```python
from build123d import *

# Parameters (mm, degrees)
SKETCH_W        = 80
SKETCH_H        = 47
PAD_DEPTH       = 4
SKETCH001_R     = 2.1
POCKET_DEPTH    = 4.001
SKETCH002_W     = 20
SKETCH002_H     = 16
PAD001_DEPTH    = 20
SKETCH003_R     = 1.6
POCKET001_DEPTH = 223.177811
POCKET002_DEPTH = 223.177811
CHAMFER_SIZE    = 3
CHAMFER_FACE9_W = 80
CHAMFER_FACE9_H = 4
POCKET003_DEPTH = 15.5
FILLET_R        = 4
FILLET001_R     = 1
SKETCH005_W     = 15
SKETCH005_H     = 16
POCKET004_DEPTH = 9
FILLET002_R     = 10


with BuildPart() as part:
    # Sketch → Pad (new body)
    with BuildSketch(Plane.XY):
        Rectangle(SKETCH_W, SKETCH_H)
    extrude(amount=PAD_DEPTH)

    # Sketch001 (on Face6 of Pad) → Pocket (cut, through all)
    with BuildSketch(Plane.XY.offset(4)):
        with Locations((-19, 19)):
            Circle(SKETCH001_R)
        with Locations((19, 19)):
            Circle(SKETCH001_R)
        with Locations((19, -19)):
            Circle(SKETCH001_R)
        with Locations((-19, -19)):
            Circle(SKETCH001_R)
    extrude(amount=-POCKET_DEPTH, mode=Mode.SUBTRACT)

    # Sketch002 (on Face5 of Pocket) → Pad001 (join)
    with BuildSketch(Plane.XY.offset(4)):
        with Locations((-30, 0)):
            Rectangle(SKETCH002_W, SKETCH002_H)
    pad001 = extrude(amount=PAD001_DEPTH)

    # Mirrored: Pad001 across YZ
    add(pad001.mirror(Plane.YZ))

    # Sketch003 (on Face15 of Mirrored) → Pocket001 (cut, through all)
    with BuildSketch(Plane.XZ.offset(8)):
        with Locations((-36, 8)):
            Circle(SKETCH003_R)
    pocket001 = extrude(amount=-POCKET001_DEPTH, mode=Mode.SUBTRACT)

    # Mirrored001: Pocket001 across YZ
    add(pocket001.mirror(Plane.YZ), mode=Mode.SUBTRACT)

    # Sketch004 (on Face15 of Mirrored001) → Pocket002 (cut, through all)
    with BuildSketch(Plane.XZ.offset(8)):
        with BuildLine():
            ThreePointArc((-40, 24), (-31.691484, 12.308516), (-20, 4))
            Line((-20, 24), (-20, 4))
            Line((-40, 24), (-20, 24))
        make_face()
    pocket002 = extrude(amount=-POCKET002_DEPTH, mode=Mode.SUBTRACT)

    # Mirrored002: Pocket002 across Sketch004 V_Axis
    add(pocket002.mirror(Plane(origin=(0, -8, 0), x_dir=(0, -1, 0), z_dir=(1, 0, 0))), mode=Mode.SUBTRACT)

    # Chamfer
    chamfer_edges = [part.edges().sort_by_distance(p)[0] for p in [
        (-40, 0, 24),
        (40, 0, 24),
    ]]
    chamfer(chamfer_edges, length=CHAMFER_SIZE)

    # Chamfer Face9 → Pocket003 (cut)
    with BuildSketch(Plane(origin=(0, -23.5, 2), x_dir=(-1, 0, 0), z_dir=(0, -1, 0))):
        Rectangle(CHAMFER_FACE9_W, CHAMFER_FACE9_H)
    extrude(amount=-POCKET003_DEPTH, mode=Mode.SUBTRACT)

    # Fillet
    fillet_edges = [part.edges().sort_by_distance(p)[0] for p in [
        (-40, 23.5, 2),
        (40, 23.5, 2),
    ]]
    fillet(fillet_edges, radius=FILLET_R)

    # Fillet001
    fillet001_edges = [part.edges().sort_by_distance(p)[0] for p in [
        (40, 13.75, 4),
    ]]
    fillet(fillet001_edges, radius=FILLET001_R)

    # Sketch005 (on DatumPlane) → Pocket004 (cut)
    with BuildSketch(Plane.XY.offset(10)):
        with Locations((-25.5, 0)):
            Rectangle(SKETCH005_W, SKETCH005_H)
    pocket004 = extrude(amount=POCKET004_DEPTH, mode=Mode.SUBTRACT)

    # Mirrored003: Pocket004 across Sketch005 V_Axis
    add(pocket004.mirror(Plane(origin=(0, 0, 10), x_dir=(0, 0, 1), z_dir=(1, 0, 0))), mode=Mode.SUBTRACT)

    # Fillet002
    fillet002_edges = [part.edges().sort_by_distance(p)[0] for p in [
        (33, 0, 13.675937),
        (29.19265, 0, 10),
        (-33, 0, 13.675937),
        (-29.19265, 0, 10),
    ]]
    fillet(fillet002_edges, radius=FILLET002_R)


solid = part.part
```
Design review of the part built by this model. Coordinates are the model's own, in mm. A direction names the side the tool comes from. Give positions to 0.01 mm unless a question says otherwise; leave off trailing zeros. Order: outer loops, then holes, each group sorted by start corner. A loop starts at its lowest first (then second) coordinate and runs counter-clockwise, first axis right, second up. Notation, with made-up numbers: (43, 31.25) - (51, 31.25) arc R7 cw to (51, 38.25) - close; hole circle Ø7 at (78.5, 55). An arc over 180 degrees is marked (long way). Use a Markdown table: item, result. Add a question column.
(1) Add section B-B on z = 11.75. Give the boundary of the cut face in (x, y), then the cut area to 3 significant figures.
(2) Machinability: for faces 1 (the face through (21.003, 19.631, 2.028)), 2 (the face through (29.51, -0.11, 9.49)), which of the approach directions +Z, -Z, +X, -X, +Y, -Y give a long, thin tool a straight path to every point of the face, cutting with its end or side? Answer none if there is none.
(3) Add section D-D on x = -16. Give the boundary of the cut face in (y, z).
(4) Mouldability with a two-part tool opening along Z and no side actions: class faces 3 (the face through (0, -8, 3)), 4 (the face through (-1, 11, 4)), 5 (the face through (-36.35, -0.11, 6.44)) as +Z half, -Z half, draft (parallel to the pull), parting line (faces both ways), or undercut.
(5) Add section C-C on y = 15. Give the boundary of the cut face in (x, z), then the cut area to 3 significant figures.
(6) Add section A-A on y = -1. Give the number of separate pieces and of enclosed holes in the cut face, then the cut area to 3 significant figures.
(7) Clearance check with flat-ended pins moving along their axes: P1, Ø2, axis at y = 8.5, z = 11, coming from the +X side; P2, Ø3.5, axis at x = 36, z = 8, coming from the +Y side; P3, Ø4, axis at x = -24, y = 20, coming from the +Z side. State where each tip first meets the part, or that it passes through.
(8) Wall thickness on probe 1 along X at (y, z) = (0.5, 8.5); probe 2 along Z at (x, y) = (36.5, 10.5); probe 3 along Y at (x, z) = (-27, 7.25): over which ranges is each line inside the solid? List them lowest first. Write a range as [from, to].
Report:
| question | item | result |
|---|---|---|
| 1 | outline | (-40, -8) - (-33.15, -8) - (-33.15, 8) - (-40, 8) - close; (33.15, -8) - (40, -8) - (40, 8) - (33.15, 8) - close |
| 1 | area | 219 mm² |
| 2 | face 1 | +Z, -Z |
| 2 | face 2 | +Z, +Y, -Y |
| 3 | outline | (-8, 0) - (23.5, 0) - (23.5, 3) arc R1 ccw to (22.5, 4) - (-8, 4) - close |
| 4 | face 3 | draft |
| 4 | face 4 | +Z half |
| 4 | face 5 | undercut |
| 5 | outline | (-40, 0) - (40, 0) - (40, 3) arc R1 ccw to (39, 4) - (-39, 4) arc R1 ccw to (-40, 3) - close |
| 5 | area | 320 mm² |
| 6 | separate pieces | 1 |
| 6 | enclosed holes | 2 |
| 6 | area | 590 mm² |
| 7 | P1 | stops at x = 40 |
| 7 | P2 | stops at y = 8 |
| 7 | P3 | stops at z = 4 |
| 8 | probe 1 | x = [-40, -37.52], [-34.48, -27.39], [27.39, 34.48], [37.52, 40] |
| 8 | probe 2 | z = [0, 4] |
| 8 | probe 3 | y = [-8, 8] |
